```python
from build123d import *

# Parameters (mm, degrees)
BASE_EXTRUDE_DEPTH = 22.225
HOLE1_REACH        = 44.241
SKETCH2_R          = 3.5687
SKETCH3_R          = 6.35
HOLE1A_DEPTH       = 40.553672
HOLE2_REACH        = 44.241
SKETCH4_R          = 3.5687
SKETCH5_R          = 6.35
HOLE2A_DEPTH       = 40.553672


with BuildPart() as part:
    # Sketch1 → Base Extrude (new body)
    with BuildSketch(Plane(origin=(0, 0, 0), x_dir=(0, 0, -1), z_dir=(1, 0, 0))):
        with BuildLine():
            Line((0, 25.4), (0, 0))
            Line((0, 0), (25.4, 0))
            Line((25.4, 0), (25.4, 2.794))
            ThreePointArc((25.4, 2.794), (25.03651, 4.62139), (24.001376, 6.170576))
            Line((24.001376, 6.170576), (6.170576, 24.001376))
            ThreePointArc((6.170576, 24.001376), (4.62139, 25.03651), (2.794, 25.4))
            Line((2.794, 25.4), (0, 25.4))
        make_face()
        with BuildLine():
            Line((4.7752, 17.41718), (4.7752, 5.2832))
            ThreePointArc((4.7752, 5.2832), (4.92399, 4.92399), (5.2832, 4.7752))
            Line((5.2832, 4.7752), (17.41718, 4.7752))
            ThreePointArc((17.41718, 4.7752), (17.88651, 5.088797), (17.77639, 5.64241))
            Line((17.77639, 5.64241), (5.64241, 17.77639))
            ThreePointArc((5.64241, 17.77639), (5.088797, 17.88651), (4.7752, 17.41718))
        make_face(mode=Mode.SUBTRACT)
    extrude(amount=-BASE_EXTRUDE_DEPTH)

    # Sketch2 → Hole1 (cut, up to next)
    with BuildSketch(Plane.XZ, mode=Mode.PRIVATE) as hole1_sk1:
        with Locations(Location((-11.1125, -12.7, 0), (0, 0, 270))):
            Circle(SKETCH2_R)
    hole1_tool1 = extrude(hole1_sk1.sketch, amount=-HOLE1_REACH, mode=Mode.PRIVATE) & part.part
    add(hole1_tool1.solids().sort_by_distance((-11.1125, 0, -12.7))[0], mode=Mode.SUBTRACT)

    # Sketch3 → Hole1a (cut, through all)
    with BuildSketch(Plane(origin=(0, 4.7752, 0), x_dir=(-1, 0, 0), z_dir=(0, 1, 0))):
        with Locations((11.1125, -12.7)):
            Circle(SKETCH3_R)
    extrude(amount=HOLE1A_DEPTH, mode=Mode.SUBTRACT)

    # Sketch4 → Hole2 (cut, up to next)
    with BuildSketch(Plane.XY, mode=Mode.PRIVATE) as hole2_sk1:
        with Locations((-11.1125, 12.7)):
            Circle(SKETCH4_R)
    hole2_tool1 = extrude(hole2_sk1.sketch, amount=-HOLE2_REACH, mode=Mode.PRIVATE) & part.part
    add(hole2_tool1.solids().sort_by_distance((-11.1125, 12.7, 0))[0], mode=Mode.SUBTRACT)

    # Sketch5 → Hole2a (cut, through all)
    with BuildSketch(Plane(origin=(0, 0, -4.7752), x_dir=(-1, 0, 0), z_dir=(0, 0, -1))):
        with Locations((11.1125, 12.7)):
            Circle(SKETCH5_R)
    extrude(amount=HOLE2A_DEPTH, mode=Mode.SUBTRACT)


solid = part.part
```
Design review of the part built by this model. Coordinates are the model's own, in mm. A direction names the side the tool comes from. Round coordinates to 2 decimals unless told otherwise and drop trailing zeros. Write each loop counter-clockwise with the first axis right and the second up, starting at its lowest first coordinate (ties: lowest second). Pieces come first, ordered by that corner, then holes. Notation, with made-up numbers: (80, 59.25) -> (113, 59.25) arc R9 cw to (113, 73.25) -> close; hole circle Ø9 at (-10.75, 15.25). An arc over 180 degrees is marked (long way). Answer in a Markdown table with one row per item.
Q1. For faces 4 (the face through (-18.42, 5.081, -17.883)), 5 (the face through (-10.939, 6.352, -19.51)), 6 (the face through (-8, 16, 0)), 7 (the face through (-13.284, 2.354, -9.868)), 8 (the face through (-11.06, 6.08, -19.05)), list the 3-axis set-ups (+Z, -Z, +X, -X, +Y, -Y) from which the entire face can be reached by the end or side of a thin tool; tool diameter is ignored.
The answers:
| item | result |
|---|---|
| face 4 | +X, -X |
| face 5 | -Z |
| face 6 | +Z, +X, -X, +Y, -Y |
| face 7 | +Y, -Y |
| face 8 | +Y |
Q2. Take a section at C-C, the plane y = 4.25. State the section outline as (x, z) points (1 decimal), then the cut area to 3 significant figures.
The answers:
| item | result |
|---|---|
| outline | (-22.2, -25.2) -> (0, -25.2) -> (0, 0) -> (-22.2, 0) -> close; hole circle Ø7.1 at (-11.1, -12.7) |
| area | 519 mm² |
Q3. Take a section at A-A, the plane x = -14. State the section outline as (y, z) points.
The answers:
| item | result |
|---|---|
| outline | (0, -25.4) -> (2.79, -25.4) arc R4.78 ccw to (6.17, -24) -> (7.04, -23.13) -> (7.04, -18.36) -> (4.78, -18.36) -> (4.78, -14.8) -> (0, -14.8) -> close; (0, -10.6) -> (4.78, -10.6) -> (4.78, -5.28) arc R0.51 cw to (5.28, -4.78) -> (10.6, -4.78) -> (10.6, 0) -> (0, 0) -> close; (14.8, -4.78) -> (18.36, -4.78) -> (18.36, -7.04) -> (23.13, -7.04) -> (24, -6.17) arc R4.78 ccw to (25.4, -2.79) -> (25.4, 0) -> (14.8, 0) -> close |
Q4. Clearance check with flat-ended pins moving along their axes: pin 1 Ø5 at (x, y) = (-12, 9) entering from -Z; pin 2 Ø1 at (x, y) = (-16.5, 22.5) entering from -Z; pin 3 Ø3 at (x, z) = (-5.5, -13.5) entering from +Y. State where each tip first meets the part, or that it passes through.
The answers:
| item | result |
|---|---|
| pin 1 | z = -4.78 |
| pin 2 | z = -8.17 |
| pin 3 | y = 17.99 |
Q5. Take a section at B-B, the plane x = -19.5. State the section outline as (y, z) points, then the cut area to 3 significant figures.
The answers:
| item | result |
|---|---|
| outline | (0, -25.4) -> (2.79, -25.4) arc R4.78 ccw to (6.17, -24) -> (24, -6.17) arc R4.78 ccw to (25.4, -2.79) -> (25.4, 0) -> (0, 0) -> close; hole (4.78, -17.42) arc R0.51 ccw to (5.64, -17.78) -> (17.78, -5.64) arc R0.51 ccw to (17.42, -4.78) -> (5.28, -4.78) arc R0.51 ccw to (4.78, -5.28) -> close |
| area | 336 mm² |
Q6. Draft analysis for pull direction X (two halves, no side actions). For faces 1 (the face through (-14.678, 12.857, -2.354)), 2 (the face through (0, 13, -13)), 3 (the face through (-10.957, 4.597, -25.046)), state which applies: +X half, -X half, draft (parallel to the pull), parting line (faces both ways), or undercut.
The answers:
| item | result |
|---|---|
| face 1 | undercut |
| face 2 | +X half |
| face 3 | draft |
Q7. To check wall thickness, follow L1, parallel to X at y = 12.7, z = -15 (1 decimal); L2, parallel to Y at x = -4.25, z = -3; L3, parallel to Y at x = -8, z = -2.5. State the ranges of each line that lie inside material, in increasing order. Write a range as [from, to].
The answers:
| item | result |
|---|---|
| L1 | [-22.2, -17.5], [-4.8, 0] |
| L2 | [0, 25.4] |
| L3 | [0, 10.95], [14.45, 25.4] |
